```python
from build123d import *

# Parameters (mm, degrees)
F0_R      = 115
F1_DEPTH  = 20
F2_R      = 115
F2_R_2    = 113.5
F3_DEPTH  = 300
F4_R      = 72
F4_R_2    = 70.5
F5_DEPTH  = 200
F6_R      = 50.5
F6_R_2    = 49
F7_DEPTH  = 150
F8_R      = 93.5
F8_R_2    = 92
F9_DEPTH  = 250
F11_DEPTH = 300
F13_DEPTH = 250
F15_DEPTH = 200
F17_DEPTH = 150


with BuildPart() as f1:
    # F0 (on Top) → F1 (new body)
    with BuildSketch(Plane.XY):
        Circle(F0_R)
    extrude(amount=F1_DEPTH)

    # F2 (on face) → F3 (join)
    with BuildSketch(Plane(origin=(0, 0, 0), x_dir=(1, 0, 0), z_dir=(0, 0, -1))):
        Circle(F2_R)
        Circle(F2_R_2, mode=Mode.SUBTRACT)
    extrude(amount=F3_DEPTH)

    # F4 (on face) → F5 (join)
    with BuildSketch(Plane(origin=(0, 0, 0), x_dir=(1, 0, 0), z_dir=(0, 0, -1))):
        Circle(F4_R)
        Circle(F4_R_2, mode=Mode.SUBTRACT)
    extrude(amount=F5_DEPTH)

    # F6 (on face) → F7 (join)
    with BuildSketch(Plane(origin=(0, 0, 0), x_dir=(1, 0, 0), z_dir=(0, 0, -1))):
        Circle(F6_R)
        Circle(F6_R_2, mode=Mode.SUBTRACT)
    extrude(amount=F7_DEPTH)

    # F8 (on face) → F9 (join)
    with BuildSketch(Plane(origin=(0, 0, 0), x_dir=(1, 0, 0), z_dir=(0, 0, -1))):
        Circle(F8_R)
        Circle(F8_R_2, mode=Mode.SUBTRACT)
    extrude(amount=F9_DEPTH)

    # F10 (on face) → F11 (cut)
    with BuildSketch(Plane(origin=(0, 0, -300), x_dir=(1, 0, 0), z_dir=(0, 0, -1))):
        with BuildLine():
            Line((-102.1050381255, -49.5662303328), (-103.3925876319, -50.3485136104))
            ThreePointArc((-103.3925876319, -50.3485136104), (0.4342578791, -114.9991800844), (103.7698839288, -49.5662303328))
            Line((103.7698839288, -49.5662303328), (102.1050381255, -49.5662303328))
            ThreePointArc((102.1050381255, -49.5662303328), (0, -113.5), (-102.1050381255, -49.5662303328))
        make_face()
    extrude(amount=-F11_DEPTH, mode=Mode.SUBTRACT)

    # F12 (on face) → F13 (cut)
    with BuildSketch(Plane(origin=(0, 0, -250), x_dir=(1, 0, 0), z_dir=(0, 0, -1))):
        with BuildLine():
            ThreePointArc((-49.3462659465, 79.4178571679), (-55.0925678888, -75.5450790152), (90.6993695659, -22.7128677261))
            Line((90.6993695659, -22.7128677261), (89.1522609902, -22.7128677261))
            ThreePointArc((89.1522609902, -22.7128677261), (-53.9825837089, -74.4975211408), (-49.3462659465, 77.6462879804))
            Line((-49.3462659465, 77.6462879804), (-49.3462659465, 79.4178571679))
        make_face()
    extrude(amount=-F13_DEPTH, mode=Mode.SUBTRACT)

    # F14 (on face) → F15 (cut)
    with BuildSketch(Plane(origin=(0, 0, -200), x_dir=(1, 0, 0), z_dir=(0, 0, -1))):
        with BuildLine():
            Line((-66.1720512268, -24.3209711245), (-67.7679154435, -24.3209711245))
            ThreePointArc((-67.7679154435, -24.3209711245), (12.3432185443, -70.9340888147), (72, 0))
            ThreePointArc((72, 0), (57.1551603856, 43.7868432442), (18.742009964, 69.5178902334))
            Line((18.742009964, 69.5178902334), (18.742009964, 67.96313017))
            ThreePointArc((18.742009964, 67.96313017), (56.0872610423, 42.713805131), (70.5, 0))
            ThreePointArc((70.5, 0), (12.3515259889, -69.4095800718), (-66.1720512268, -24.3209711245))
        make_face()
    extrude(amount=-F15_DEPTH, mode=Mode.SUBTRACT)

    # F16 (on face) → F17 (cut)
    with BuildSketch(Plane(origin=(0, 0, -150), x_dir=(1, 0, 0), z_dir=(0, 0, -1))):
        with BuildLine():
            ThreePointArc((50.5, 0), (0, 50.5), (-50.5, 0))
            Line((-50.5, 0), (-49, 0))
            ThreePointArc((-49, 0), (0, 49), (49, 0))
            Line((49, 0), (50.5, 0))
        make_face()
    extrude(amount=-F17_DEPTH, mode=Mode.SUBTRACT)


solid = f1.part
```
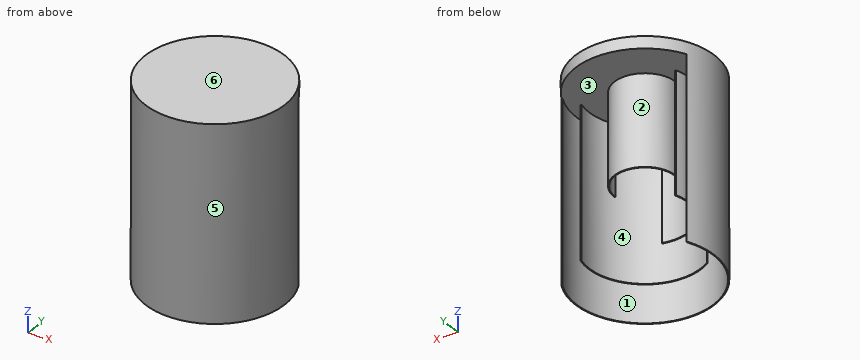
Could you check a few things on this model? Use its own coordinates, in mm. Face numbers are marked on the shaded views. A direction names the side the tool comes from. Give positions to 0.01 mm unless a question says otherwise; leave off trailing zeros. Write each loop counter-clockwise with the first axis right and the second up, starting at its lowest first coordinate (ties: lowest second). Pieces come first, ordered by that corner, then holes. Notation, with made-up numbers: (1.25, 10) -> (31.25, 10) arc R24 cw to (31.25, 24) -> close; hole circle Ø8 at (12.25, -38). An arc over 180 degrees is marked (long way). Write each question's results on one line, items separated by ' | '.
1. I need wall thicknesses on L1, parallel to Y at x = 0, z = -64; L2, parallel to Y at x = 0, z = -196.5; L3, parallel to X at y = 0, z = -232. Which ranges of each line are inside material? Lowest first, please.
Check sheet entries:
L1: y = -115 to -113.5, -93.5 to -92, -72 to -70.5, 49 to 50.5 | L2: y = -115 to -113.5, -93.5 to -92, -72 to -70.5 | L3: x = -115 to -113.5, 92 to 93.5, 113.5 to 115
2. I want a section at C-C, the plane x = 0. Write out the boundary of the cut face in (y, z).
Check sheet entries:
outline: (-115, -300) -> (-113.5, -300) -> (-113.5, 0) -> (-93.5, 0) -> (-93.5, -250) -> (-92, -250) -> (-92, 0) -> (-72, 0) -> (-72, -200) -> (-70.5, -200) -> (-70.5, 0) -> (49, 0) -> (49, -150) -> (50.5, -150) -> (50.5, 0) -> (115, 0) -> (115, 20) -> (-115, 20) -> close
3. On a 3-axis mill with a long thin cutter (end or side, diameter ignored), from which of +Z, -Z, +X, -X, +Y, -Y can I reach the whole of each face in a straight line? I mean the marked faces 1 and 2. Say none if no direction works.
Check sheet entries:
face 1: -Z | face 2: -Z, +Y
4. I want a section at B-B, the plane z = -22. Write out the boundary of the cut face in (x, y).
Check sheet entries:
outline: (-103.39, 50.35) arc R115 ccw (long way) to (103.77, 49.57) -> (102.11, 49.57) arc R113.5 cw (long way) to (-102.11, 49.57) -> close; (-67.77, 24.32) arc R72 ccw to (18.74, -69.52) -> (18.74, -67.96) arc R70.5 cw to (-66.17, 24.32) -> close; (-50.5, 0) -> (-49, 0) arc R49 cw to (49, 0) -> (50.5, 0) arc R50.5 ccw to start; (-49.35, -79.42) arc R93.5 ccw to (90.7, 22.71) -> (89.15, 22.71) arc R92 cw to (-49.35, -77.65) -> close
5. If we mould it in two halves opening along X, with no side actions, what happens to the marked faces 3, 4, 5 and 6? For each: released by +X, released by -X, zero draft, split by the parting line, or undercut.
Check sheet entries:
face 3: undercut | face 4: undercut | face 5: split by the parting line | face 6: zero draft
6. I want a section at A-A, the plane z = -190. Write out the boundary of the cut face in (x, y).
Check sheet entries:
outline: (-103.39, 50.35) arc R115 ccw (long way) to (103.77, 49.57) -> (102.11, 49.57) arc R113.5 cw (long way) to (-102.11, 49.57) -> close; (-67.77, 24.32) arc R72 ccw to (18.74, -69.52) -> (18.74, -67.96) arc R70.5 cw to (-66.17, 24.32) -> close; (-49.35, -79.42) arc R93.5 ccw to (90.7, 22.71) -> (89.15, 22.71) arc R92 cw to (-49.35, -77.65) -> close
7. Will these pins go through, and if not, where does the flat tip stop? pin 1 Ø1.3 at (x, z) = (103.5, -132) entering from +Y; pin 2 Ø0.9 at (y, z) = (-78, -154.5) entering from -X; pin 3 Ø2 at (y, z) = (-69, -121) entering from +X.
Check sheet entries:
pin 1: stops at y = 49.57 | pin 2: stops at x = -84.92 | pin 3: stops at x = 92.74
8. I want a section at D-D, the plane y = 36. Write out the boundary of the cut face in (x, z).
Check sheet entries:
outline: (-109.22, -300) -> (-107.64, -300) -> (-107.64, 0) -> (-35.42, 0) -> (-35.42, -150) -> (-33.24, -150) -> (-33.24, 0) -> (33.24, 0) -> (33.24, -150) -> (35.42, -150) -> (35.42, 0) -> (107.64, 0) -> (107.64, -300) -> (109.22, -300) -> (109.22, 20) -> (-109.22, 20) -> close
